Can you work these out from the model? Positions are in its coordinate system, mm. Face numbers are marked on the shaded views. A direction names the side the tool comes from. Round coordinates to 2 decimals unless told otherwise and drop trailing zeros. Write each loop counter-clockwise with the first axis right and the second up, starting at its lowest first coordinate (ties: lowest second). Pieces come first, ordered by that corner, then holes. Notation, with made-up numbers: M 26.5,60 L 81.5,60 A21 ccw 81.5,72 Z; hole C 31,21.5 d2. An arc over 180 degrees is marked long. Answer as a JSON object with one key per item and string values. Group by question number.
1) I'm going to push flat-ended pins straight in: pin 1 Ø4 at (x, y) = (-9.5, -7.5) entering from -Z; pin 2 Ø2 at (x, z) = (1.5, 5.5) entering from +Y; pin 3 Ø5 at (x, z) = (-8.5, 3.5) entering from +Y; pin 4 Ø3 at (y, z) = (2.5, 4.5) entering from -X. Where does each tip first touch, or does it pass through?
2) Suppose I cut it at A-A, the plane y = 0. Write out the boundary of the cut face in (x, z), and give its area (3 significant figures).
3) On a 3-axis mill with a long thin cutter (end or side, diameter ignored), from which of +Z, -Z, +X, -X, +Y, -Y can I reach the whole of each face in a straight line? I mean the marked faces 4 and 5. Say none if no direction works.
4) Suppose I cut it at B-B, the plane x = -9.75. Write out the boundary of the cut face in (y, z).
5) If we mould it in two halves opening along Z, with no side actions, what happens to the marked faces 1, 2 and 3? For each: +Z half, -Z half, draft (parallel to the pull), parting line (faces both ways), or undercut.
6) Suppose I cut it at D-D, the plane z = 12.5. Write out the boundary of the cut face in (x, y), and give its area (3 significant figures).
7) Please list where these lines run through material, in increasing order: L1, parallel to Z at x = -7.5, y = -0.25; L2, parallel to Y at x = -9, z = 4.5; L3, parallel to Y at x = -6.25, z = 3.75. Write a range as [from, to].
8) Suppose I cut it at C-C, the plane z = 2. Write out the boundary of the cut face in (x, y), and give its area (3 significant figures).
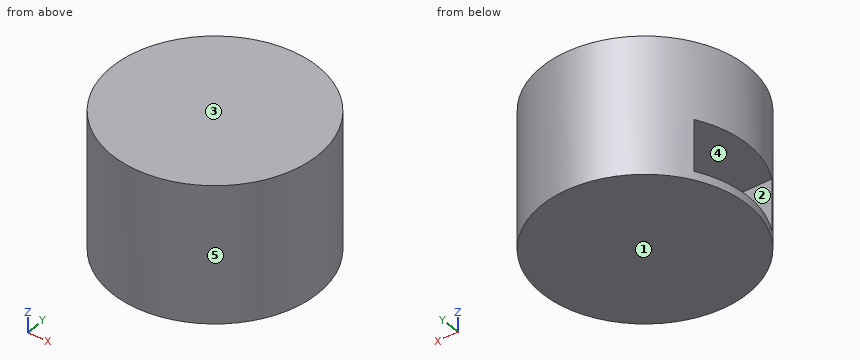
from build123d import *

# Parameters (mm, degrees)
CROQUIS1_R                 = 12
SALIENTE_EXTRUIR1_DEPTH    = 16
CORTAR_EXTRUIR1_DEPTH      = 1
CORTAR_EXTRUIR1_DEPTH_BACK = 9
CROQUIS3_W                 = 6
CROQUIS3_H                 = 12


with BuildPart() as part:
    # Croquis1 → Saliente-Extruir1 (new body)
    with BuildSketch(Plane.XY):
        Circle(CROQUIS1_R)
    extrude(amount=SALIENTE_EXTRUIR1_DEPTH)

    # Croquis3 → Cortar-Extruir1 (cut, two sides: drawn at the far end of the back side and taken through both)
    with BuildSketch(Plane.ZY.offset(12).offset(-CORTAR_EXTRUIR1_DEPTH_BACK)):
        with Locations((4, 0)):
            Rectangle(CROQUIS3_W, CROQUIS3_H)
    extrude(amount=CORTAR_EXTRUIR1_DEPTH + CORTAR_EXTRUIR1_DEPTH_BACK, mode=Mode.SUBTRACT)


solid = part.part
Results:
{
 "1": {"pin 1": "z = 0", "pin 2": "y = 11.99", "pin 3": "y = 10.39", "pin 4": "x = -3"},
 "2": {"outline": "M -12,0 L 12,0 L 12,16 L -12,16 L -12,7 L -3,7 L -3,1 L -12,1 Z", "area": "330 mm^2"},
 "3": {"face 4": "-X", "face 5": "+Z, -Z"},
 "4": {"outline": "M -7,0 L 7,0 L 7,16 L -7,16 Z; hole M -6,1 L 6,1 L 6,7 L -6,7 Z"},
 "5": {"face 1": "-Z half", "face 2": "undercut", "face 3": "+Z half"},
 "6": {"outline": "C 0,0 d24", "area": "452 mm^2"},
 "7": {"L1": "[0, 1], [7, 16]", "L2": "[-7.94, -6], [6, 7.94]", "L3": "[-10.24, -6], [6, 10.24]"},
 "8": {"outline": "M -10.39,-6 A12 ccw long -10.39,6 L -3,6 L -3,-6 Z", "area": "351 mm^2"}
}
